Geometry: final body of the model. Coordinates: model frame, mm. Face numbers are marked on the shaded views. A direction names the side the tool comes from. Give positions to 0.01 mm unless a question says otherwise; leave off trailing zeros. Loops run counter-clockwise (first coordinate to the right, second up) from the corner with the lowest first, then second, coordinate; pieces in that order, holes last. Notation, with made-up numbers: (0.25, 53.25) - (54.25, 53.25) arc R24 cw to (54.25, 66.25) - close; hole circle Ø10 at (33.5, 18). An arc over 180 degrees is marked (long way). Answer in a Markdown table with one row per item.
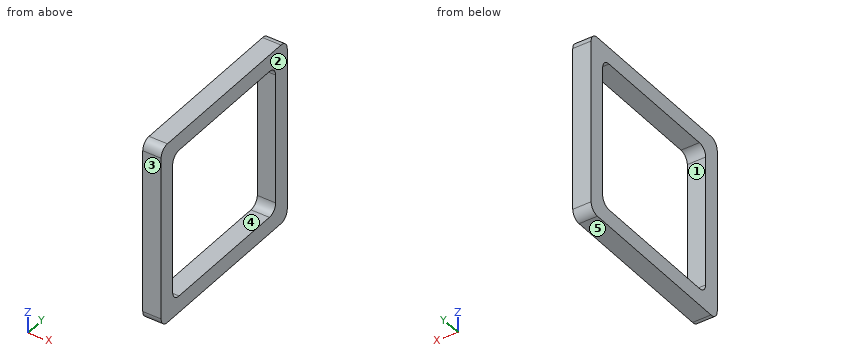
from build123d import *

# Parameters (mm, degrees)
SKETCH1_W           = 31.75
SKETCH1_H           = 31.75
SKETCH1_W_2         = 25.908
SKETCH1_H_2         = 25.908
BOSS_EXTRUDE1_DEPTH = 1.5875
FILLET1_R           = 1.5875


with BuildPart() as part:
    # Sketch1 → Boss-Extrude1 (new, symmetric)
    with BuildSketch(Plane(origin=(0, 0, 0), x_dir=(0, 0, -1), z_dir=(1, 0, 0))):
        with Locations((15.875, 15.875)):
            Rectangle(SKETCH1_W, SKETCH1_H)
        with Locations((15.875, 15.875)):
            Rectangle(SKETCH1_W_2, SKETCH1_H_2, mode=Mode.SUBTRACT)
    extrude(amount=BOSS_EXTRUDE1_DEPTH, both=True)

    # Fillet1
    fillet1_edges = [part.edges().sort_by_distance(p)[0] for p in [
        (0, 2.921, -2.921),
        (0, 2.921, -28.829),
        (0, 28.829, -28.829),
        (0, 28.829, -2.921),
        (0, 31.75, 0),
        (0, 31.75, -31.75),
        (0, 0, -31.75),
        (0, 0, 0),
    ]]
    fillet(fillet1_edges, radius=FILLET1_R)


solid = part.part
Q1. Cut plane B-B (y = 10). Output: boundary loops of the cut face in (x, z), and give its area (3 significant figures).
Check values:
| item | result |
|---|---|
| outline | (-1.59, -31.75) - (1.59, -31.75) - (1.59, -28.83) - (-1.59, -28.83) - close; (-1.59, -2.92) - (1.59, -2.92) - (1.59, 0) - (-1.59, 0) - close |
| area | 18.5 mm² |
Q2. Reachability of the marked faces 4 and 5 from +Z, -Z, +X, -X, +Y, -Y: full face, straight path, thin tool, end or side. Return the list, or none.
Check values:
| item | result |
|---|---|
| face 4 | +X, -X |
| face 5 | -Z, +X, -X, +Y, -Y |
Q3. Material intervals for line 1 along Z through (x, y) = (-0.15, 18); line 2 along Y through (x, z) = (1.3, -17); line 3 along Z through (x, y) = (0.2, 28.5), sorted ascending.
Check values:
| item | result |
|---|---|
| line 1 | -31.75 to -28.83, -2.92 to 0 |
| line 2 | 0 to 2.92, 28.83 to 31.75 |
| line 3 | -31.75 to -28.21, -3.54 to 0 |
Q4. Cut plane C-C (z = -26). Output: boundary loops of the cut face in (x, y), and give its area (3 significant figures).
Check values:
| item | result |
|---|---|
| outline | (-1.59, 0) - (1.59, 0) - (1.59, 2.92) - (-1.59, 2.92) - close; (-1.59, 28.83) - (1.59, 28.83) - (1.59, 31.75) - (-1.59, 31.75) - close |
| area | 18.5 mm² |
Q5. Draft query along Y for the marked faces 1, 2 and 3. Return one class per face: pulls with the +Y half, pulls with the -Y half, needs draft (parallel to the pull), parting line crosses it, or undercut.
Check values:
| item | result |
|---|---|
| face 1 | undercut |
| face 2 | needs draft |
| face 3 | pulls with the -Y half |
